from build123d import *

# Parameters (mm, degrees)
SKETCH_1_W          = 228.6
SKETCH_1_H          = 5
EXTRUDE_1_DEPTH     = 55.99999976
SKETCH_2_R          = 15
CUT_EXTRUDE_1_DEPTH = 28
SKETCH_3_W          = 228.6
SKETCH_3_H          = 6.022861395
EXTRUDE_2_DEPTH     = 22.666
SKETCH_4_W          = 2.077402036
SKETCH_4_H          = 55.99999976
SKETCH_4_W_2        = 2.004864202
EXTRUDE_3_DEPTH     = 22.412
EXTRUDE_4_DEPTH     = 6.156
CUT_EXTRUDE_2_DEPTH = 6.156


with BuildPart() as part:
    # 草图1 → 凸台-拉伸1 (new body)
    with BuildSketch(Plane.XY):
        with Locations((-114.3, 2.5)):
            Rectangle(SKETCH_1_W, SKETCH_1_H)
    extrude(amount=EXTRUDE_1_DEPTH)

    # 草图2 → 切除-拉伸1 (cut)
    with BuildSketch(Plane(origin=(0, 5, 0), x_dir=(1, 0, 0), z_dir=(0, 1, 0))):
        with Locations(Location((-210.039051384, -27.99999988, 0), (0, 0, 180))):
            Circle(SKETCH_2_R)
        with Locations(Location((-171.783646654, -27.99999988, 0), (0, 0, 180))):
            Circle(SKETCH_2_R)
        with Locations(Location((-133.528241924, -27.99999988, 0), (0, 0, 180))):
            Circle(SKETCH_2_R)
        with Locations(Location((-95.272837194, -27.99999988, 0), (0, 0, 180))):
            Circle(SKETCH_2_R)
        with Locations(Location((-57.017432464, -27.99999988, 0), (0, 0, 180))):
            Circle(SKETCH_2_R)
        with Locations(Location((-18.762027734, -27.99999988, 0), (0, 0, 180))):
            Circle(SKETCH_2_R)
    extrude(amount=-CUT_EXTRUDE_1_DEPTH, mode=Mode.SUBTRACT)

    # 草图3 → 凸台-拉伸2 (add)
    with BuildSketch(Plane(origin=(0, 5, 0), x_dir=(1, 0, 0), z_dir=(0, 1, 0))):
        with Locations((-114.3, -3.011430698)):
            Rectangle(SKETCH_3_W, SKETCH_3_H)
    extrude(amount=EXTRUDE_2_DEPTH)

    # 草图4 → 凸台-拉伸3 (add)
    with BuildSketch(Plane.XZ):
        with Locations((-227.561298982, 27.99999988)):
            Rectangle(SKETCH_4_W, SKETCH_4_H)
        with Locations((-1.002432101, 27.99999988)):
            Rectangle(SKETCH_4_W_2, SKETCH_4_H)
    extrude(amount=EXTRUDE_3_DEPTH)

    # 草图5 → 凸台-拉伸4 (add)
    with BuildSketch(Plane.XZ.offset(22.412)):
        Polygon((-228.6, 55.99999976), (-228.6, 0), (-226.522597964, 0), (84.340152487, 0), (84.340152487, 55.99999976), (-226.522597964, 55.99999976), align=None)
    extrude(amount=EXTRUDE_4_DEPTH)

    # 草图7 → 切除-拉伸2 (cut)
    with BuildSketch(Plane.XZ.offset(28.568)):
        with BuildLine():
            Line((12.810419977, 31.513278328), (72.336600875, 31.513278328))
            ThreePointArc((72.336600875, 31.513278328), (75.849879323, 27.99999988), (72.336600875, 24.486721432))
            Line((72.336600875, 24.486721432), (12.810419977, 24.486721432))
            ThreePointArc((12.810419977, 24.486721432), (9.297141529, 27.99999988), (12.810419977, 31.513278328))
        make_face()
    extrude(amount=-CUT_EXTRUDE_2_DEPTH, mode=Mode.SUBTRACT)


solid = part.part
For this review, take the finished solid that the model builds, in its own axes (mm). A direction names the side the tool comes from. Round coordinates to 2 decimals unless told otherwise and drop trailing zeros. Loops run counter-clockwise (first coordinate to the right, second up) from the corner with the lowest first, then second, coordinate; pieces in that order, holes last. Notation, with made-up numbers: (39.25, 33.5) - (67.25, 33.5) arc R19 cw to (67.25, 68.5) - close; hole circle Ø4 at (-7.75, 65.5). An arc over 180 degrees is marked (long way). One line per question, with ' | ' between items.
Q1. For pin 1 (24 mm diameter, centred on x = -57.02, z = 28, fed in from +Y); pin 2 (5 mm diameter, centred on x = 39, y = -24.5, fed in from -Z); pin 3 (8 mm diameter, centred on y = 11, z = 20, fed in from -X); pin 4 (17 mm diameter, centred on x = -79.5, z = 33.5, fed in from +Y), all flat-tipped, find the tip position at first contact; note any pin that passes through.
Taken from the geometry:
pin 1: stops at y = -22.41 | pin 2: stops at z = 0 | pin 3: passes through | pin 4: stops at y = 5
Q2. Take a section at A-A (y = -12). Give the boundary of the cut face in (x, z), and give its area (3 significant figures).
Taken from the geometry:
outline: (-228.6, 0) - (-226.52, 0) - (-226.52, 56) - (-228.6, 56) - close; (-2, 0) - (0, 0) - (0, 56) - (-2, 56) - close | area: 229 mm²
Q3. Take a section at B-B (x = -189.5). Give the boundary of the cut face in (y, z).
Taken from the geometry:
outline: (-28.57, 0) - (-22.41, 0) - (-22.41, 56) - (-28.57, 56) - close; (0, 0) - (27.67, 0) - (27.67, 6.02) - (5, 6.02) - (5, 56) - (0, 56) - close
Q4. Tool access review of faces 4 (the flat face through (-226.523, -11, 28)), 5 (the cylindrical face through (75.85, -25.53, 28.08)), 6 (the cylindrical face through (-70.87, 2.54, 22.25)): name each direction out of +Z, -Z, +X, -X, +Y, -Y from which nothing blocks a thin tool from reaching the whole face with its end or side.
Taken from the geometry:
face 4: +Z, -Z | face 5: +Y, -Y | face 6: +Y
Q5. For line 1 along X through (y, z) = (-8, 39); line 2 along Y through (x, z) = (-121.5, 46); line 3 along Y through (x, z) = (18, 13), list the stretches that pass through material, from the lowest coordinate up. Write a range as [from, to].
Taken from the geometry:
line 1: x = [-228.6, -226.52], [-2, 0] | line 2: y = [-28.57, -22.41], [0, 5] | line 3: y = [-28.57, -22.41]
Q6. Take a section at D-D (z = 52). Give the boundary of the cut face in (x, y), and give its area (3 significant figures).
Taken from the geometry:
outline: (-228.6, -28.57) - (84.34, -28.57) - (84.34, -22.41) - (0, -22.41) - (0, 5) - (-228.6, 5) - close; hole (-226.52, -22.41) - (-2, -22.41) - (-2, 0) - (-226.52, 0) - close | area: 3,160 mm²
Q7. Take a section at C-C (z = 38.5). State how many separate pieces and enclosed holes the cut face has, and give its area (3 significant figures).
Taken from the geometry:
separate pieces: 6 | enclosed holes: 0 | area: 2,520 mm²
Q8. The part is to be moulded in two halves that separate along Z. For faces 1 (the flat face through (-116, 27.666, 3)), 2 (the flat face through (-109, 6, 0)), 3 (the flat face through (42, -26, 31.513)), say which applies: released by +Z, released by -Z, zero draft, split by the parting line, or undercut.
Taken from the geometry:
face 1: zero draft | face 2: released by -Z | face 3: undercut
